Can you work these out from the model? Positions are in its coordinate system, mm. A direction names the side the tool comes from. Round coordinates to 2 decimals unless told otherwise and drop trailing zeros. Loops run counter-clockwise (first coordinate to the right, second up) from the corner with the lowest first, then second, coordinate; pieces in that order, holes last. Notation, with made-up numbers: M 9.5,63.25 L 22.5,63.25 A19 cw 22.5,91.25 Z; hole C 4.5,80 d9. An arc over 180 degrees is marked long. Return JSON: item names as keys, results as strings.
Autodesk Inventor part; units mm, degrees
ref_plane "YZ Plane" through (0, 0, 0) normal (1, 0, 0) x (0, 1, 0)
ref_plane "XZ Plane" through (0, 0, 0) normal (0, 1, 0) x (-1, 0, 0)
ref_plane "XY Plane" through (0, 0, 0) normal (0, 0, 1) x (1, 0, 0)
sketch "Sketch2" plane through (0, 0, 0) normal (0, 0, 1) x (1, 0, 0)
  circle A0 centre (3.2039, 4.4261) radius 14.1
  circle A1 centre (3.2039, 4.4261) radius 12.1
  line L0 (-1.7961, -8.7576) -> (8.2039, -8.7576)
  line L1 (-1.7961, -8.7576) -> (-1.7961, -9.7576)
  line L2 (-1.7961, -9.7576) -> (8.2039, -9.7576)
  line L3 (8.2039, -9.7576) -> (8.2039, -8.7576)
  line L4 (-8.8961, 4.4261) -> (-10.8961, 4.4261)
  line L5 (15.3039, 4.4261) -> (17.3039, 4.4261)
  dimension "d6" = 28.2
  dimension "d7" = 24.2
  dimension "d8" = 1
  dimension "d9" = 10
extrude "Extrusion2" add sketch "Sketch2" along normal blind 10 contours A0 L0 L4 A1 L5 | L3 L2 L1 A0 | A0 L0
properties part number "clip-pipe" material "PC/ABS Plastic"
Q1. Suppose I cut it at A-A, the plane y = -3.5. Please give me the cut outline in (x, z), plus the area to 3 significant figures.
Results:
{"outline": "M -8.46,0 L -5.94,0 L -5.94,10 L -8.46,10 Z; M 12.35,0 L 14.87,0 L 14.87,10 L 12.35,10 Z", "area": "50.4 mm2"}
Q2. I'm going to push flat-ended pins straight in: pin 1 Ø0.8 at (y, z) = (-9, 4.5) entering from -X; pin 2 Ø4 at (x, z) = (2, 8) entering from +Y; pin 3 Ø1.5 at (x, z) = (-8, 3) entering from -Y. Where does each tip first touch, or does it pass through?
Results:
{"pin 1": "stops at x = -2.19", "pin 2": "stops at y = -7.24", "pin 3": "stops at y = -5.04"}
Q3. Suppose I cut it at D-D, the plane x = 13.5. Please give me the cut outline in (y, z), plus the area to 3 significant figures.
Results:
{"outline": "M -5.21,0 L -1.93,0 L -1.93,10 L -5.21,10 Z", "area": "32.8 mm2"}
Q4. If I drill on line 1 along Y through (x, z) = (3, 2.25); line 2 along X through (y, z) = (-5.5, 7.5); line 3 along X through (y, z) = (-6, 6), over which ranges is the centre line in solid material (lowest first)?
Results:
{"line 1": "y = -9.76 to -7.67", "line 2": "x = -6.81 to -3.72, 10.12 to 13.22", "line 3": "x = -6.29 to -2.94, 9.34 to 12.7"}
Q5. On a 3-axis mill with a long thin cutter (end or side, diameter ignored), from which of +Z, -Z, +X, -X, +Y, -Y can I reach the whole of each face in a straight line? I mean faces 1 (the flat face through (-1.796, -9, 5)), 2 (the flat face through (3, -8, 0)), 3 (the flat face through (8.204, -9, 5)). Say none if no direction works.
Results:
{"face 1": "+Z, -Z, -X, -Y", "face 2": "-Z, +X, -X, +Y, -Y", "face 3": "+Z, -Z, +X, -Y"}
Q6. Suppose I cut it at C-C, the plane y = 1. Please give me the cut outline in (x, z).
Results:
{"outline": "M -10.47,0 L -8.4,0 L -8.4,10 L -10.47,10 Z; M 14.81,0 L 16.88,0 L 16.88,10 L 14.81,10 Z"}
Q7. Suppose I cut it at B-B, the plane z = 1.75. Please give me the cut outline in (x, y).
Results:
{"outline": "M -10.9,4.43 A14.1 ccw -1.8,-8.76 L -1.8,-9.76 L 8.2,-9.76 L 8.2,-8.76 A14.1 ccw 17.3,4.43 L 15.3,4.43 A12.1 cw -8.9,4.43 Z"}
